```python
from build123d import *

# Parameters (mm, degrees)
FILLET1_R = 0.5


with BuildPart() as part:
    # Sketch2 → Revolve1 (revolve)
    with BuildSketch(Plane.XY):
        with BuildLine():
            Line((-86.101123841, -5.64973336), (-88.101123841, -5.64973336))
            Line((-88.101123841, -5.64973336), (-89.278275677, -5.64973336))
            ThreePointArc((-89.278275677, -5.64973336), (-89.10084359, -0.391604097), (-88.569354565, 4.842603093))
            ThreePointArc((-88.569354565, 4.842603093), (-87.443565623, 6.803114863), (-85.26891575, 7.421099549))
            ThreePointArc((-85.26891575, 7.421099549), (-80.518231075, 7.223948348), (-75.784663044, 7.672509564))
            ThreePointArc((-75.784663044, 7.672509564), (-73.546078322, 7.850154417), (-71.309016698, 7.654260207))
            ThreePointArc((-71.309016698, 7.654260207), (-66.960113272, 6.937963646), (-62.601123841, 6.28584947))
            Line((-62.601123841, 6.28584947), (-62.601123841, 5.275841234))
            ThreePointArc((-62.601123841, 5.275841234), (-67.04517898, 5.939067763), (-71.478802412, 6.668779202))
            ThreePointArc((-71.478802412, 6.668779202), (-81.654724965, 3.910052669), (-86.101123841, -5.64973336))
        make_face()
    revolve(axis=Axis((86.398876159, -5.64973336, 0), (-1, 0, 0)))

    # Fillet1
    # the kernel refuses this fillet: 0.5 mm, written as the material it takes off along each edge
    with BuildSketch(Plane(origin=(-62.601123841, -5.64973336, 0), x_dir=(0, 1, 0), z_dir=(0, 0, 1))) as fillet1_piece_1:
        with BuildLine():
            CenterArc((11.501916817, 0.5), FILLET1_R, 270, 81.83079423)
            ThreePointArc((11.99684319, 0.428951526), (11.966135307, 0.21448686), (11.93558283, 0))
            Line((11.93558283, 0), (11.501916817, 0))
        make_face()
    revolve(axis=Axis((-62.601123841, -5.64973336, 0), (-1, 0, 0)), mode=Mode.SUBTRACT)
    with BuildSketch(Plane(origin=(-62.601123841, -5.64973336, 0), x_dir=(0, 1, 0), z_dir=(0, 0, 1))) as fillet1_piece_2:
        with BuildLine():
            CenterArc((11.501916817, 0.5), FILLET1_R, 171.83079423, 98.16920577)
            ThreePointArc((11.006990445, 0.571048474), (10.966145272, 0.285543805), (10.925574594, 0))
            Line((10.925574594, 0), (11.501916817, 0))
        make_face()
    revolve(axis=Axis((-62.601123841, -5.64973336, 0), (-1, 0, 0)), mode=Mode.SUBTRACT)


solid = part.part
```
Design review of the part built by this model. Coordinates are the model's own, in mm. Give positions to 0.01 mm unless a question says otherwise; leave off trailing zeros. Loops run counter-clockwise (first coordinate to the right, second up) from the corner with the lowest first, then second, coordinate; pieces in that order, holes last. Notation, with made-up numbers: (2, -28.5) -> (38, -28.5) arc R21 cw to (38, -7.5) -> close; hole circle Ø6 at (-27, 34). An arc over 180 degrees is marked (long way). One line per item, written item: value.
Q1. For pin 1 Ø5 at (x, y) = (-83, 5) entering from -Z; pin 2 Ø10 at (y, z) = (4, 0) entering from -X; pin 3 Ø10 at (x, y) = (-77.5, -16) entering from +Z, all flat-tipped, find the tip position at first contact; note any pin that passes through.
Numbers:
pin 1: stops at z = -10
pin 2: stops at x = -89.14
pin 3: stops at z = 12.06
Q2. For L1, parallel to Z at x = -66, y = -1.25; L2, parallel to Z at x = -73.5, y = 2; L3, parallel to Y at x = -69.75, z = 6, list the stretches that pass through material, from the lowest coordinate up.
Numbers:
L1: z = -11.63 to -10.55, 10.55 to 11.63
L2: z = -11.12 to -9.89, 9.89 to 11.12
L3: y = -17.23 to -16.07, 4.77 to 5.93
Q3. We need section A-A on x = -84.5. Give the boundary of the cut face in (y, z).
Numbers:
outline: circle Ø25.99 at (-5.65, 0); hole circle Ø12.24 at (-5.65, 0)
